Verification items for the finished model (mm, model axes). Face numbers are marked on the shaded views. A direction names the side the tool comes from. Coordinates: 2 decimals unless noted, no trailing zeros. Order: outer loops, then holes, each group sorted by start corner. A loop starts at its lowest first (then second) coordinate and runs counter-clockwise, first axis right, second up. Notation, with made-up numbers: M -22.5,20 L -17.5,20 A29 cw -17.5,58 Z; hole C 54.5,-10 d3. An arc over 180 degrees is marked long. Return JSON: item names as keys, results as strings. Group by question number.
Q1. Section check C-C, the plane z = -9. Enter the section's corners in (x, y).
Q2. Section check B-B, the plane z = 40. Enter the section's corners in (x, y), then the cut area to 3 significant figures.
Q3. Thickness scan on probe 1 along Z at (x, y) = (0, 0); probe 2 along Z at (x, y) = (-17.5, -10); probe 3 along X at (y, z) = (-12.5, 23). Record the ranges inside material, lowest first.
Q4. Mould release check, pull along Z, two halves, no side actions. Record for the marked faces 4, 5, 6 and 7: pulls with the +Z half, pulls with the -Z half, needs draft (parallel to the pull), parting line crosses it, or undercut.
Q5. Go/stop test with flat-tipped pins: pin 1 Ø8 at (x, z) = (10.5, -21.5) entering from -Y; pin 2 Ø2 at (x, y) = (12.5, -18) entering from -Z; pin 3 Ø4 at (x, z) = (10.5, 17.5) entering from -Y; pin 4 Ø5 at (x, z) = (-9, 7) entering from +Y. Record where each tip stops, or that it passes through.
Q6. Access from +Z, -Z, +X, -X, +Y, -Y to the whole of each face (thin tool, end or side, straight path). Record for the marked faces 1, 2 and 3.
from build123d import *

# Parameters (mm, degrees)
F0_R     = 25
F1_DEPTH = 50
F2_W     = 10
F2_H     = 20
F3_DEPTH = 40
F6_R     = 9.99999
F7_R     = 5
F5_D     = 10


# Not quite as in the source:
# - a fillet or chamfer is up to 0.001 mm smaller than in the source, because OpenCascade refuses the exact size


with BuildPart() as f1:
    # F0 (on Top) → F1 (new body)
    with BuildSketch(Plane.XY):
        Circle(F0_R)
    extrude(amount=F1_DEPTH)

    # F2 (on face) → F3 (join)
    with BuildSketch(Plane(origin=(0, 0, 0), x_dir=(1, 0, 0), z_dir=(0, 0, -1))):
        Rectangle(F2_W, F2_H)
    extrude(amount=F3_DEPTH)

    # F6 (radius 10 in the source; OpenCascade refuses exactly that, so slightly less here)
    f6_edges = [f1.edges().sort_by_distance(p)[0] for p in [
        (0, 10, -40),
        (0, -10, -40),
    ]]
    fillet(f6_edges, radius=F6_R)

    # F7
    f7_edges = [f1.edges().sort_by_distance(p)[0] for p in [
        (-25, 0, 50),
        (-25, 0, 0),
        (-5, 0, 0),
        (0, -10, 0),
        (5, 0, 0),
        (0, 10, 0),
    ]]
    fillet(f7_edges, radius=F7_R)

    # F5 (through all)
    with Locations(Plane(origin=(-5, 0, 0), x_dir=(0, -1, 0), z_dir=(-1, 0, 0))):
        with Locations((0, -30)):
            Hole(F5_D / 2)


solid = f1.part
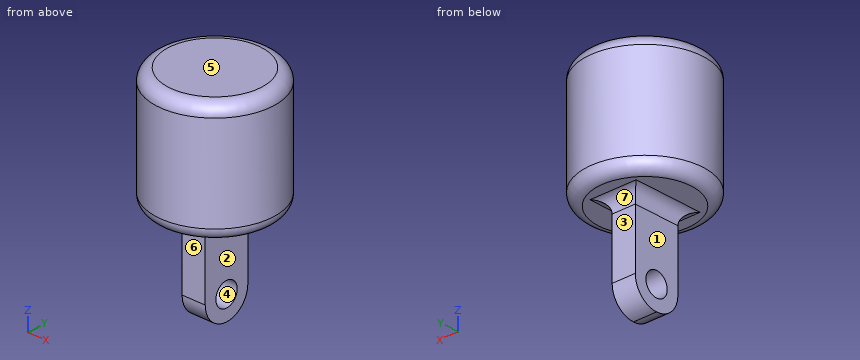
Numbers:
{
 "1": {"outline": "M -5,-10 L 5,-10 L 5,10 L -5,10 Z"},
 "2": {"outline": "C 0,0 d50", "area": "1,960 mm2"},
 "3": {"probe 1": "z = -40 to -35, -25 to 50", "probe 2": "z = 0 to 50", "probe 3": "x = -21.65 to 21.65"},
 "4": {"face 4": "undercut", "face 5": "pulls with the +Z half", "face 6": "needs draft", "face 7": "pulls with the -Z half"},
 "5": {"pin 1": "passes through", "pin 2": "stops at z = 0.08", "pin 3": "stops at y = -23.51", "pin 4": "stops at y = 24.14"},
 "6": {"face 1": "-Z, -X, +Y, -Y", "face 2": "-Z, +X, +Y, -Y", "face 3": "-Z, +X, -X, +Y"}
}
